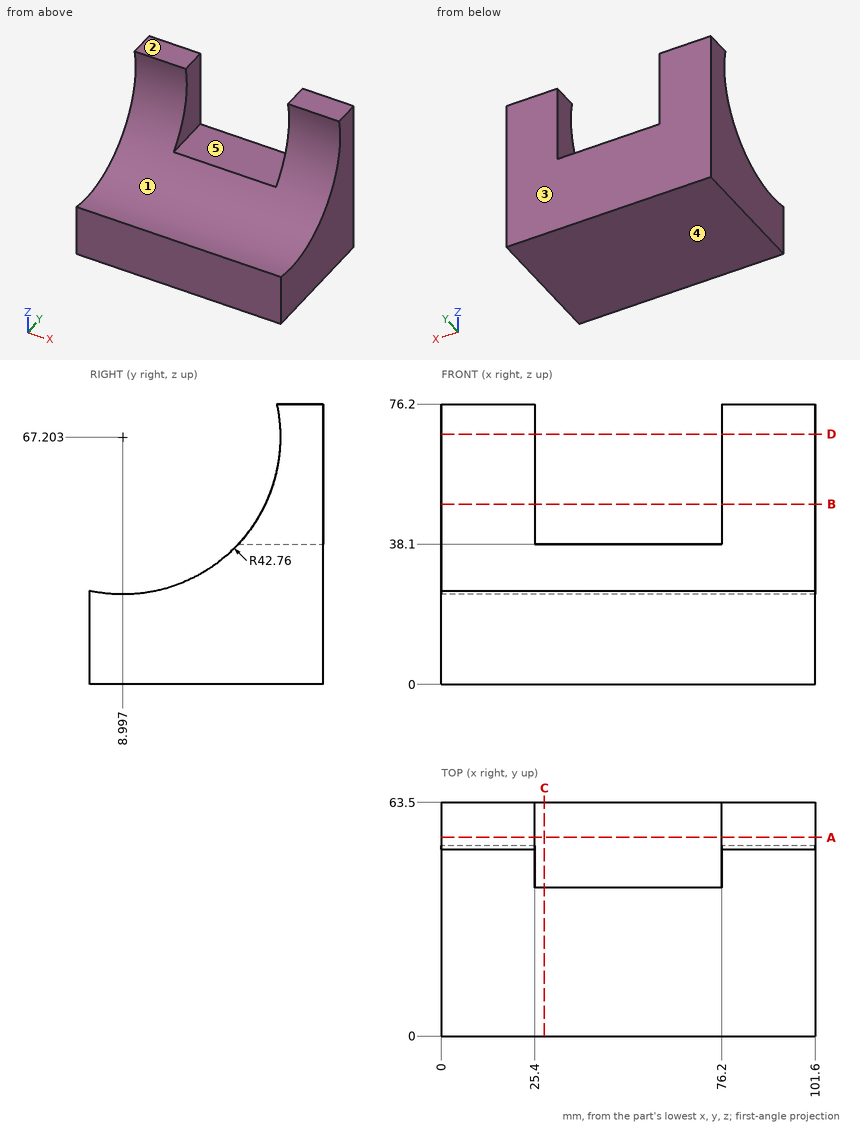
Here's the drawing with two shaded views (mm, measured from the low corner). I have some questions. A direction names the side the tool comes from. Give positions to 0.01 mm unless a question says otherwise; leave off trailing zeros. Order: outer loops, then holes, each group sorted by start corner. A loop starts at its lowest first (then second) coordinate and runs counter-clockwise, first axis right, second up. Notation, with made-up numbers: M 65,8 L 100,8 A25 cw 100,45 Z; hole C 28,-10.75 d10. An arc over 180 degrees is marked long. One line per item, written item: value.
1) I want a section at B-B, the plane z = 49. List the corners of the cut face in (x, y) for me.
Answer sheet:
outline: M 0,47.69 L 25.4,47.69 L 25.4,63.5 L 0,63.5 Z; M 76.2,47.69 L 101.6,47.69 L 101.6,63.5 L 76.2,63.5 Z
2) I want a section at A-A, the plane y = 54. List the corners of the cut face in (x, z) for me.
Answer sheet:
outline: M 0,0 L 101.6,0 L 101.6,76.2 L 76.2,76.2 L 76.2,38.1 L 25.4,38.1 L 25.4,76.2 L 0,76.2 Z
3) I want a section at D-D, the plane z = 68. List the corners of the cut face in (x, y) for me, plus the area to 3 significant figures.
Answer sheet:
outline: M 0,51.75 L 25.4,51.75 L 25.4,63.5 L 0,63.5 Z; M 76.2,51.75 L 101.6,51.75 L 101.6,63.5 L 76.2,63.5 Z
area: 597 mm^2
4) Please list where these lines run through material, in increasing order: line 1 along X through (y, z) = (61.5, 62.5); line 2 along Y through (x, z) = (83, 71); line 3 along Z through (x, y) = (38.5, 44.5).
Answer sheet:
line 1: x = 0 to 25.4, 76.2 to 101.6
line 2: y = 51.59 to 63.5
line 3: z = 0 to 38.1
5) On a 3-axis mill with a long thin cutter (end or side, diameter ignored), from which of +Z, -Z, +X, -X, +Y, -Y can I reach the whole of each face in a straight line? I mean the marked faces 4 and 5. Say none if no direction works.
Answer sheet:
face 4: -Z, +X, -X, +Y, -Y
face 5: +Z, +Y, -Y
6) We'd pull the mould along Z, two halves only. Please class the marked faces 1, 2 and 3: released by +Z, released by -Z, zero draft, split by the parting line, or undercut.
Answer sheet:
face 1: undercut
face 2: released by +Z
face 3: zero draft
7) For P1, Ø10, axis at x = 58.5, z = 16, coming from the -Y side; P2, Ø7, axis at x = 55.5, y = 56.5, coming from the +Z side; P3, Ø8, axis at x = 24, z = 67.5, coming from the -Y side; P4, Ø5, axis at x = 75.5, y = 8.5, coming from the +Z side, each with a flat end and sliding along its axis, tell me the tip position at first contact or that it passes through.
Answer sheet:
P1: stops at y = 0
P2: stops at z = 38.1
P3: stops at y = 51.54
P4: stops at z = 24.55
8) I want a section at C-C, the plane x = 28. List the corners of the cut face in (y, z) for me (1 decimal), plus the area to 3 significant figures.
Answer sheet:
outline: M 0,0 L 63.5,0 L 63.5,38.1 L 40.3,38.1 A42.8 cw 0,25.4 Z
area: 2,000 mm^2
